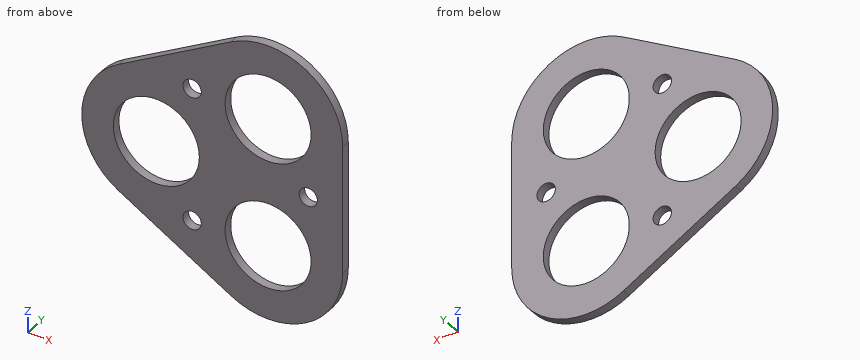
from build123d import *

# Parameters (mm, degrees)
SKETCH1_R           = 7.5
SKETCH1_R_2         = 1.6
SKETCH1_R_3         = 1.599999998
BOSS_EXTRUDE1_DEPTH = 1.5


with BuildPart() as part:
    # Sketch1 → Boss-Extrude1 (new body)
    with BuildSketch(Plane(origin=(0, 0, 0), x_dir=(1, 0, 0), z_dir=(0, 1, 0))):
        with BuildLine():
            Line((-15.804326324, -11.258330249), (3.681245261, -22.508330249))
            ThreePointArc((3.681245261, -22.508330249), (16.681245261, -22.508330249), (23.181245261, -11.25))
            Line((23.181245261, -11.25), (23.181245261, 11.25))
            ThreePointArc((23.181245261, 11.25), (16.681245261, 22.508330249), (3.681245261, 22.508330249))
            Line((3.681245261, 22.508330249), (-15.804326324, 11.258330249))
            ThreePointArc((-15.804326324, 11.258330249), (-22.304326324, 0), (-15.804326324, -11.258330249))
        make_face()
        with Locations((-9.304326324, 0)):
            Circle(SKETCH1_R, mode=Mode.SUBTRACT)
        with Locations((-3.06154027, 11.687177858)):
            Circle(SKETCH1_R_2, mode=Mode.SUBTRACT)
        with Locations((17.181245264, 0)):
            Circle(SKETCH1_R_3, mode=Mode.SUBTRACT)
        with Locations((10.181245261, -11.25)):
            Circle(SKETCH1_R, mode=Mode.SUBTRACT)
        with Locations((10.181245261, 11.25)):
            Circle(SKETCH1_R, mode=Mode.SUBTRACT)
        with Locations((-3.06154027, -11.687177373)):
            Circle(SKETCH1_R_2, mode=Mode.SUBTRACT)
    extrude(amount=BOSS_EXTRUDE1_DEPTH)


solid = part.part
Part model, mm, in its own coordinate system. Coordinates: 2 decimals unless noted, no trailing zeros. Write each loop counter-clockwise with the first axis right and the second up, starting at its lowest first coordinate (ties: lowest second). Pieces come first, ordered by that corner, then holes. Notation, with made-up numbers: M 46,-6 L 57,-6 A6 ccw 57,4 Z; hole C 61,16.5 d10. An arc over 180 degrees is marked long. Return JSON: item names as keys, results as strings.
1. Saw through at B-B, the plane x = -5.5. Write the cut outline in (y, z).
Determined:
{"outline": "M 0,-17.21 L 1.5,-17.21 L 1.5,-6.46 L 0,-6.46 Z; M 0,6.46 L 1.5,6.46 L 1.5,17.21 L 0,17.21 Z"}
2. Saw through at C-C, the plane x = 13.5. Write the cut outline in (y, z).
Determined:
{"outline": "M 0,-23.82 L 1.5,-23.82 L 1.5,-17.98 L 0,-17.98 Z; M 0,-4.52 L 1.5,-4.52 L 1.5,4.52 L 0,4.52 Z; M 0,17.98 L 1.5,17.98 L 1.5,23.82 L 0,23.82 Z"}
3. Saw through at D-D, the plane y = 0.4. Write the cut outline in (x, z), then the cut area to 3 significant figures.
Determined:
{"outline": "M -15.8,-11.26 L 3.68,-22.51 A13 ccw 23.18,-11.25 L 23.18,11.25 A13 ccw 3.68,22.51 L -15.8,11.26 A13 ccw Z; hole C -9.3,0 d15; hole C -3.06,-11.69 d3.2; hole C -3.06,11.69 d3.2; hole C 10.18,-11.25 d15; hole C 10.18,11.25 d15; hole C 17.18,0 d3.2", "area": "1,070 mm²"}
4. Flat gauge pin, fed straight in: pin 1 Ø17 at (x, z) = (10.18, -11.25) entering from -Y. Where does the tip first touch, or does it go through?
Determined:
{"pin 1": "y = 0"}
5. Probe L1, parallel to X at y = 0.3, z = 11.25; L2, parallel to X at y = 0.3, z = 4.5; L3, parallel to Z at x = 4.5, y = 0.7. List the from-to ranges inside material, lowest first.
Determined:
{"L1": "-15.82 to -4.6, -1.52 to 2.68, 17.68 to 23.18", "L2": "-21.5 to -15.3, -3.3 to 6.91, 13.45 to 23.18", "L3": "-22.94 to -16.15, -6.35 to 6.35, 16.15 to 22.94"}
6. Saw through at A-A, the plane z = 0. Write the cut outline in (x, y).
Determined:
{"outline": "M -22.3,0 L -16.8,0 L -16.8,1.5 L -22.3,1.5 Z; M -1.8,0 L 15.58,0 L 15.58,1.5 L -1.8,1.5 Z; M 18.78,0 L 23.18,0 L 23.18,1.5 L 18.78,1.5 Z"}
